Part print with two shaded views. Sizes in mm from the minimum x, y, z corner. A direction names the side the tool comes from. Round coordinates to 2 decimals unless told otherwise and drop trailing zeros. Loops run counter-clockwise (first coordinate to the right, second up) from the corner with the lowest first, then second, coordinate; pieces in that order, holes last. Notation, with made-up numbers: M 61.5,68 L 102.5,68 A24 ccw 102.5,102 Z; hole C 21,-13.75 d2. An arc over 180 degrees is marked long. Answer as CSV lines item,"result". Start each with the question number.
Item 1: Band-saw the part on C-C (x = 13). Give the cut face in (y, z) (1 decimal), and give its area (3 significant figures).
Item 2: Wall check: line 1 (Y direction, x = 40, z = 85.5); line 2 (Y direction, x = 40, z = 103); line 3 (Y direction, x = 48, z = 88.5) (1 decimal). Give the ranges that are in metal, low to high.
Item 3: Mould opens along Y. For the marked faces 1, 2 and 3 say: pulls with the +Y half, pulls with the -Y half, needs draft (parallel to the pull), parting line crosses it, or undercut.
Item 4: Which spindle directions (+Z, -Z, +X, -X, +Y, -Y) get a long thin tool onto all of the face, cutting with end or side? Do the marked faces 4, 5 and 6. Say none if no direction does.
Item 5: Drop flat-ended pins along their axis: pin 1 Ø3 at (x, y) = (38.5, 165.5) entering from -Z; pin 2 Ø4 at (x, z) = (26.5, 106) entering from -Y; pin 3 Ø6 at (x, z) = (49, 66.5) entering from -Y (1 decimal). Give the stop position or say it passes through.
Item 6: Band-saw the part on D-D (y = 208). Give the cut face in (x, z).
Item 7: Band-saw the part on A-A (x = 40). Give the cut face in (y, z).
Item 8: Band-saw the part on B-B (y = 46.5). Give the cut face in (x, z), and give its area (3 significant figures).
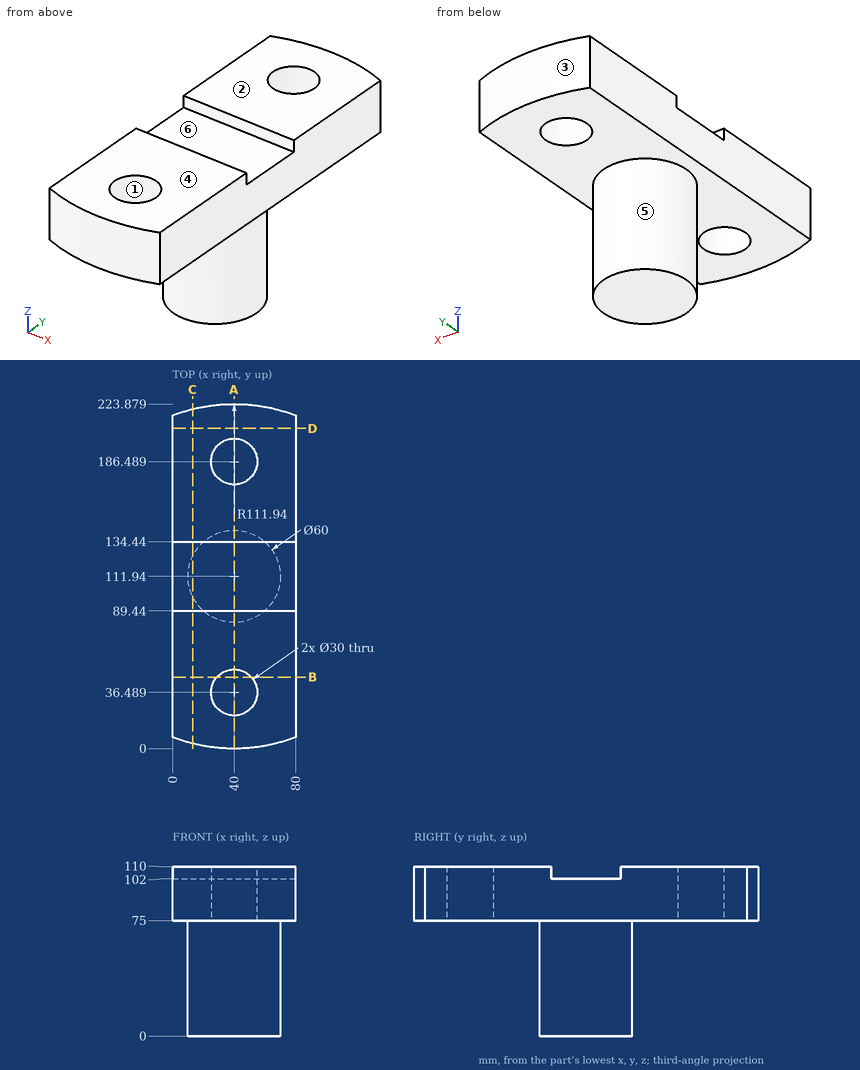
Answer block:
1,outline,"M 3.3,75 L 98.9,75 L 98.9,0 L 125,0 L 125,75 L 220.6,75 L 220.6,110 L 134.4,110 L 134.4,102 L 89.4,102 L 89.4,110 L 3.3,110 Z"
1,area,"9,210 mm^2"
2,line 1,"y = 0 to 21.49, 51.49 to 171.49, 201.49 to 223.88"
2,line 2,"y = 0 to 21.49, 51.49 to 89.44, 134.44 to 171.49, 201.49 to 223.88"
2,line 3,"y = 0.3 to 23.8, 49.2 to 173.8, 199.2 to 223.6"
3,face 1,"undercut"
3,face 2,"needs draft"
3,face 3,"pulls with the +Y half"
4,face 4,"+Z, +X, -X, +Y, -Y"
4,face 5,"-Z"
4,face 6,"+Z, +X, -X"
5,pin 1,"stops at z = 75"
5,pin 2,"stops at y = 0.59"
5,pin 3,"stops at y = 82.5"
6,outline,"M 0,75 L 80,75 L 80,110 L 0,110 Z"
7,outline,"M 0,75 L 21.49,75 L 21.49,110 L 0,110 Z; M 51.49,75 L 81.94,75 L 81.94,0 L 141.94,0 L 141.94,75 L 171.49,75 L 171.49,110 L 134.44,110 L 134.44,102 L 89.44,102 L 89.44,110 L 51.49,110 Z; M 201.49,75 L 223.88,75 L 223.88,110 L 201.49,110 Z"
8,outline,"M 0,75 L 28.83,75 L 28.83,110 L 0,110 Z; M 51.17,75 L 80,75 L 80,110 L 51.17,110 Z"
8,area,"2,020 mm^2"
